Geometry check sheet. Reference: the model listing, model coordinates, mm. Coordinates: 2 decimals unless noted, no trailing zeros. Write each loop counter-clockwise with the first axis right and the second up, starting at its lowest first coordinate (ties: lowest second). Pieces come first, ordered by that corner, then holes. Notation, with made-up numbers: (85.5, 89.5) -> (102.5, 89.5) arc R36 ccw to (102.5, 126.5) -> close; hole circle Ø10 at (71, 63). An arc over 180 degrees is marked (long way). Answer in a Markdown table with one row per item. Add a question column.
1. Cross-section at C-C on z = -10. Record the cut outline in (x, y), and give its area (3 significant figures).
2. Scan lines: L1, parallel to X at y = 1.2, z = -10; L2, parallel to Z at x = 10, y = 1.35; L3, parallel to Z at x = 134, y = 2.8. Record each from-to range of solid material in increasing order. Write a range as from..to.
3. Depth check by flat-ended pin: P1, Ø0.9, axis at x = 12, y = 1.5, coming from the +Z side; P2, Ø0.9, axis at y = 1, z = 3, coming from the +X side; P3, Ø5.5, axis at x = 10, z = -10, coming from the +Y side. Enter the tip coordinate at first touch or a pass-through.
4. Cross-section at B-B on z = 2. Record the cut outline in (x, y).
5. Cross-section at D-D on y = 0.9. Record the cut outline in (x, z).
6. Cross-section at A-A on x = 10. Record the cut outline in (y, z), and give its area (3 significant figures).
```python
from build123d import *

# Parameters (mm, degrees)
SKETCH1_R           = 3
BOSS_EXTRUDE1_DEPTH = 3


with BuildPart() as part:
    # Sketch1 → Boss-Extrude1 (new body)
    with BuildSketch(Plane(origin=(0, 0, 0), x_dir=(1, 0, 0), z_dir=(0, 1, 0))):
        Polygon((0, 0), (19, 0), (19, -3.9), (39, -3.9), (39, 0), (129, 0), (129, -3.9), (149, -3.9), (149, 0), (168, 0), (168, 20), (0, 20), align=None)
        with Locations((10, 10)):
            Circle(SKETCH1_R, mode=Mode.SUBTRACT)
        with BuildLine():
            Line((158, 7), (98, 7))
            ThreePointArc((98, 7), (95, 10), (98, 13))
            Line((98, 13), (158, 13))
            ThreePointArc((158, 13), (161, 10), (158, 7))
        make_face(mode=Mode.SUBTRACT)
    extrude(amount=BOSS_EXTRUDE1_DEPTH)


solid = part.part
```
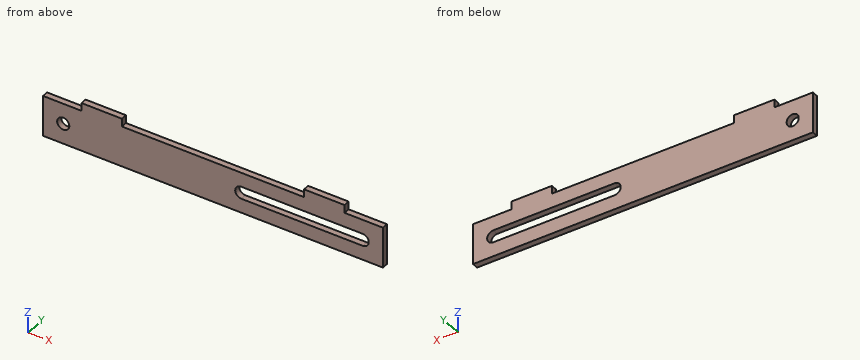
Results found:
| question | item | result |
|---|---|---|
| 1 | outline | (0, 0) -> (7, 0) -> (7, 3) -> (0, 3) -> close; (13, 0) -> (95, 0) -> (95, 3) -> (13, 3) -> close; (161, 0) -> (168, 0) -> (168, 3) -> (161, 3) -> close |
| 1 | area | 288 mm^2 |
| 2 | L1 | x = 0..7, 13..95, 161..168 |
| 2 | L2 | z = -20..-13, -7..0 |
| 2 | L3 | z = -20..-13, -7..3.9 |
| 3 | P1 | stops at z = 0 |
| 3 | P2 | stops at x = 149 |
| 3 | P3 | passes through |
| 4 | outline | (19, 0) -> (39, 0) -> (39, 3) -> (19, 3) -> close; (129, 0) -> (149, 0) -> (149, 3) -> (129, 3) -> close |
| 5 | outline | (0, -20) -> (168, -20) -> (168, 0) -> (149, 0) -> (149, 3.9) -> (129, 3.9) -> (129, 0) -> (39, 0) -> (39, 3.9) -> (19, 3.9) -> (19, 0) -> (0, 0) -> close; hole circle Ø6 at (10, -10); hole (98, -13) -> (158, -13) arc R3 ccw to (158, -7) -> (98, -7) arc R3 ccw to start |
| 6 | outline | (0, -20) -> (3, -20) -> (3, -13) -> (0, -13) -> close; (0, -7) -> (3, -7) -> (3, 0) -> (0, 0) -> close |
| 6 | area | 42.0 mm^2 |
